The model under review builds one solid part; all positions refer to its coordinate system, in mm. A direction names the side the tool comes from. Give positions to 0.01 mm unless a question says otherwise; leave off trailing zeros. Loops run counter-clockwise (first coordinate to the right, second up) from the corner with the lowest first, then second, coordinate; pieces in that order, holes last. Notation, with made-up numbers: M -35,48.25 L -4,48.25 A12 cw -4,61.25 Z; hole C 18.25,5 d11. An arc over 180 degrees is marked long. Write item = value, one per line. Start each with the question number.
1. For faces 1 (the face through (-18, -1, 15.5)), 2 (the face through (-15.5, 10, 14)), 3 (the face through (-18.5, 10.8, 14.8)), list the 3-axis set-ups (+Z, -Z, +X, -X, +Y, -Y) from which the entire face can be reached by the end or side of a thin tool; tool diameter is ignored.
2. For pin 1 (2 mm diameter, centred on x = -15, z = 12, fed in from +Y); pin 2 (3 mm diameter, centred on x = -17, z = 14.5, fed in from -Y); pin 3 (2.5 mm diameter, centred on x = -17.74, y = 3.06, fed in from +Z); pin 4 (1.5 mm diameter, centred on x = -17, z = 16, fed in from +Y), all flat-tipped, find the tip position at first contact; note any pin that passes through.
3. Wall thickness on line 1 along Y through (x, z) = (-18.5, 16) (3 decimals); line 2 along Z through (x, y) = (-18, 5.75); line 3 along X through (y, z) = (12, 10.5): over which ranges is each line inside the solid? List them lowest first. Write a range as from..to.
4. We need section C-C on z = 16.75. Give the boundary of the cut face in (x, y), then the cut area to 3 significant figures.
5. We need section D-D on x = -17.5. Give the boundary of the cut face in (y, z).
6. We need section A-A on y = 2. Give the boundary of the cut face in (x, z).
7. We need section B-B on x = -16.5. Give the boundary of the cut face in (y, z).
8. Draft analysis for pull direction X (two halves, no side actions). For faces 4 (the face through (-18.542, 7.544, 17.844)), 5 (the face through (-14.547, -6.744, 16.768)), 6 (the face through (-16.14, 3.13, 16.73)), 7 (the face through (-18.57, 14.02, 9.78)), state which applies: pulls with the +X half, pulls with the -X half, needs draft (parallel to the pull), parting line crosses it, or undercut.
from build123d import *

# Parameters (mm, degrees)
SKETCH_4_R           = 4.196960071
EXTRUDE_3_DEPTH      = 0.6
EXTRUDE_START        = 0.6
SKETCH_5_R           = 4.196960071
EXTRUDE_4_DEPTH      = 0.6
SKETCH_8_R           = 1.6
EXTRUDE_6_DEPTH      = 2.5
SKETCH_9_R           = 27.5
EXTRUDE_7_DEPTH      = 2.5
SKETCH_10_W          = 6
SKETCH_10_H          = 20
CUT_EXTRUDE_1_DEPTH  = 49.812552895
CUT_EXTRUDE_8_DEPTH  = 49.812552895
CUT_EXTRUDE_9_DEPTH  = 6
CUT_EXTRUDE_START    = -31.2
SKETCH_19_R          = 4.196960071
CUT_EXTRUDE_10_DEPTH = 31.2
SKETCH_20_R          = 1.6
CUT_EXTRUDE_11_DEPTH = 40.445330411
FILLET_1_R           = 2


with BuildPart() as part:
    # ｽｹｯﾁ1 → 回転1 (revolve)
    with BuildSketch(Plane(origin=(0, 0, 0), x_dir=(1, 0, 0), z_dir=(0, -0.7071067811865488, 0.7071067811865464)), mode=Mode.PRIVATE) as revolve_1_sk:
        with BuildLine():
            Line((-22.696960071, 15), (-18.5, 15))
            Line((-18.5, 15), (-18.5, -15))
            Line((-18.5, -15), (-22.696960071, -15))
            ThreePointArc((-22.696960071, -15), (-25, 0), (-22.696960071, 15))
        make_face()
    revolve(revolve_1_sk.sketch.rotate(Axis((-18.5, 17.67766953, 17.67766953), (0, -0.7071067811865462, -0.7071067811865488)), 270), axis=Axis((-18.5, 17.67766953, 17.67766953), (0, -0.7071067811865462, -0.7071067811865488)))

    # ｽｹｯﾁ4 → ﾎﾞｽ - 押し出し3 (add)
    with BuildSketch(Plane(origin=(0, -10.606601718, -10.606601718), x_dir=(1, 0, 0), z_dir=(0, -0.7071067811865462, -0.7071067811865488))):
        with Locations(Location((-18.5, 0, 0), (0, 0, 90))):
            Circle(SKETCH_4_R)
    extrude(amount=EXTRUDE_3_DEPTH)

    # ｽｹｯﾁ5 → ﾎﾞｽ - 押し出し4 (add)
    with BuildSketch(Plane(origin=(0, 10.606601718, 10.606601718), x_dir=(1, 0, 0), z_dir=(0, 0.7071067811865462, 0.7071067811865488)).offset(EXTRUDE_START)):
        with Locations(Location((-18.5, 0, 0), (0, 0, 270))):
            Circle(SKETCH_5_R)
    extrude(amount=-EXTRUDE_4_DEPTH)

    # ｽｹｯﾁ8 → ﾎﾞｽ - 押し出し6 (add)
    with BuildSketch(Plane(origin=(0, 11.030865787, 11.030865787), x_dir=(1, 0, 0), z_dir=(0, 0.7071067811865462, 0.7071067811865488))):
        with BuildLine():
            Line((-15.5, -9.999999662), (-21.5, -9.999999662))
            Line((-21.5, -9.999999662), (-21.5, 3.38e-07))
            ThreePointArc((-21.5, 3.38e-07), (-18.5, 3), (-15.5, 3.38e-07))
            Line((-15.5, 3.38e-07), (-15.5, -9.999999662))
        make_face()
        with Locations(Location((-18.5, 0, 0), (0, 0, 270))):
            Circle(SKETCH_8_R, mode=Mode.SUBTRACT)
    extrude(amount=EXTRUDE_6_DEPTH)

    # ｽｹｯﾁ9 → ﾎﾞｽ - 押し出し7 (add)
    with BuildSketch(Plane.XY.offset(18)):
        Circle(SKETCH_9_R)
    extrude(amount=-EXTRUDE_7_DEPTH)

    # ｽｹｯﾁ10 → ｶｯﾄ - 押し出し1 (cut, through all)
    with BuildSketch(Plane(origin=(0, 0, 15.5), x_dir=(-1, 0, 0), z_dir=(0, 0, -1))):
        with Locations((24.5, 0.097265479)):
            Rectangle(SKETCH_10_W, SKETCH_10_H)
    extrude(amount=-CUT_EXTRUDE_1_DEPTH, mode=Mode.SUBTRACT)

    # ｽｹｯﾁ16 → ｶｯﾄ - 押し出し8 (cut, through all)
    with BuildSketch(Plane(origin=(0, 0, 15.5), x_dir=(-1, 0, 0), z_dir=(0, 0, -1))):
        with BuildLine():
            Line((25.579195254, 10.097265479), (15.5, 10.097265479))
            Line((15.5, 10.097265479), (15.5, 22.715633383))
            ThreePointArc((15.5, 22.715633383), (21.486760408, 17.163016261), (25.579195254, 10.097265479))
        make_face()
    extrude(amount=-CUT_EXTRUDE_8_DEPTH, mode=Mode.SUBTRACT)

    # ｽｹｯﾁ17 → ｶｯﾄ - 押し出し9 (cut)
    with BuildSketch(Plane.ZY.offset(21.5)):
        Polygon((15.5, 10.097265479), (18, 10.097265479), (19.869700312, 5.727565167), (18.101933359, 3.959798214), (18, 4.061731573), (18, 7.597265479), align=None)
    extrude(amount=-CUT_EXTRUDE_9_DEPTH, mode=Mode.SUBTRACT)

    # ｽｹｯﾁ19 → ｶｯﾄ - 押し出し10 (cut)
    with BuildSketch(Plane(origin=(0, -11.030865787, -11.030865787), x_dir=(1, 0, 0), z_dir=(0, -0.7071067811865462, -0.7071067811865488)).offset(CUT_EXTRUDE_START)):
        with Locations((-18.5, 0)):
            Circle(SKETCH_19_R)
    extrude(amount=CUT_EXTRUDE_10_DEPTH, mode=Mode.SUBTRACT)


with BuildPart() as body_2:
    # of the pieces the cut leaves, the one that is kept (cut_extrude_10_keep)
    add(part.part.solids().sort_by_distance((-21.5, 6.561731573, 15.5))[0])

    # ｽｹｯﾁ20 → ｶｯﾄ - 押し出し11 (cut, through all)
    with BuildSketch(Plane(origin=(0, 0, 15.5), x_dir=(-1, 0, 0), z_dir=(0, 0, -1))):
        with Locations((17.73769432, 3.061731573)):
            Circle(SKETCH_20_R)
        with Locations((17.564365692, -3.936122183)):
            Circle(SKETCH_20_R)
        with BuildLine():
            Line((21.5, 6.561731573), (19.802086592, -7.435049061))
            Line((19.802086592, -7.435049061), (13.802086592, -7.435049061))
            Line((13.802086592, -7.435049061), (15.5, 6.561731573))
            Line((15.5, 6.561731573), (15.5, 22.715633383))
            ThreePointArc((15.5, 22.715633383), (-26.256917644, -8.174611664), (25.655132995, -9.902734521))
            Line((25.655132995, -9.902734521), (21.5, -9.902734521))
            Line((21.5, -9.902734521), (21.5, 6.561731573))
        make_face()
    extrude(amount=-CUT_EXTRUDE_11_DEPTH, mode=Mode.SUBTRACT)

    # ﾌｨﾚｯﾄ1
    fillet_1_edges = [body_2.edges().sort_by_distance(p)[0] for p in [
        (-18.5, 6.561731573, 15.5),
        (-18.5, 7.597265479, 18),
        (-13.802086592, -7.435049061, 16.75),
        (-19.802086592, -7.435049061, 16.75),
    ]]
    fillet(fillet_1_edges, radius=FILLET_1_R)


solid = body_2.part
Final values:
q1.face_1 = -Z, +X, -X, -Y
q1.face_2 = +Z, -Z, +X, +Y
q1.face_3 = +Z, +X, -X, +Y
q2.pin_1 = 13.91
q2.pin_2 = -7.44
q2.pin_3 = through
q2.pin_4 = 10.35
q3.line_1 = -7.379..-5.234, -2.638..1.655, 4.468..9.597
q3.line_2 = 15.5..18
q3.line_3 = -21.31..-19.7, -17.3..-15.69
q4.outline = M -21.5,6.56 L -20.02,-5.68 A2 ccw -18.03,-7.44 L -16.06,-7.44 A2 ccw -14.07,-5.19 L -15.5,6.56 L -15.5,8.85 L -21.5,8.85 Z; hole C -17.74,3.06 d3.2; hole C -17.56,-3.94 d3.2
q4.area = 79.8 mm²
q5.outline = M -7.44,15.5 L -5.53,15.5 L -5.53,18 L -7.44,18 Z; M -2.34,15.5 L 1.48,15.5 L 1.48,18 L -2.34,18 Z; M 4.64,15.5 L 5.73,15.5 A2 cw 7.15,14.91 L 10.15,11.91 L 11.92,13.68 L 8.18,17.41 A2 ccw 6.77,18 L 4.64,18 Z; M 11.91,10.15 L 13.03,9.03 L 14.8,10.8 L 13.68,11.92 Z
q6.outline = M -20.95,15.5 L -18.93,15.5 L -18.93,18 L -20.95,18 Z; M -16.54,15.5 L -14.95,15.5 L -14.95,18 L -16.54,18 Z
q7.outline = M -7.44,15.5 L -5.13,15.5 L -5.13,18 L -7.44,18 Z; M -2.74,15.5 L 2.05,15.5 L 2.05,18 L -2.74,18 Z; M 4.08,15.5 L 5.73,15.5 A2 cw 7.15,14.91 L 12.61,9.45 L 14.38,11.22 L 8.18,17.41 A2 ccw 6.77,18 L 4.08,18 Z
q8.face_4 = needs draft
q8.face_5 = pulls with the +X half
q8.face_6 = undercut
q8.face_7 = parting line crosses it
